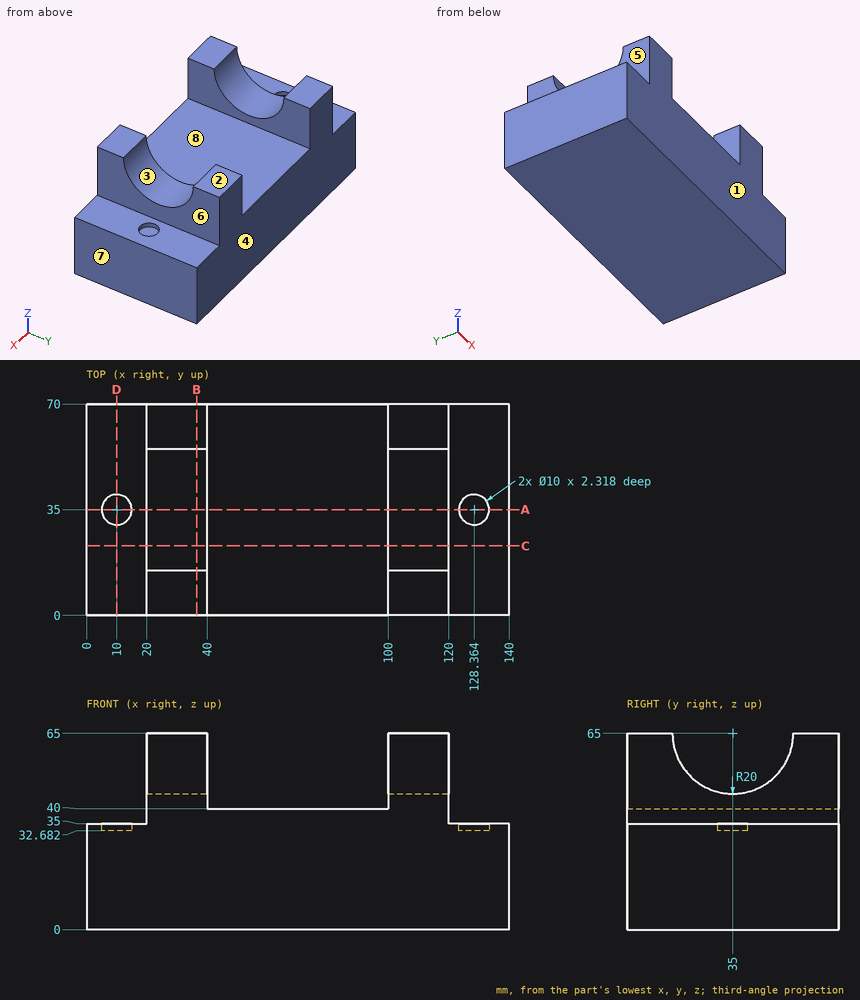
Here's the drawing with two shaded views (mm, measured from the low corner). I have some questions. A direction names the side the tool comes from. Round coordinates to 2 decimals unless told otherwise and drop trailing zeros. Write each loop counter-clockwise with the first axis right and the second up, starting at its lowest first coordinate (ties: lowest second). Pieces come first, ordered by that corner, then holes. Notation, with made-up numbers: M 50,50 L 71,50 A32 ccw 71,82 Z; hole C 4,69.5 d10. An arc over 180 degrees is marked long. Answer in a Markdown table with one row per item. Add a question column.
Q1. On a 3-axis mill with a long thin cutter (end or side, diameter ignored), from which of +Z, -Z, +X, -X, +Y, -Y can I reach the whole of each face in a straight line? I mean the marked faces 5, 6, 7 and 8. Say none if no direction works.
Q2. Imagine slicing it at A-A (y = 35). Please give me the cut outline in (x, z), then the cut area to 3 significant figures.
Q3. If we mould it in two halves opening along Y, with no side actions, what happens to the marked faces 1, 2, 3 and 4? For each: +Y half, -Y half, draft (parallel to the pull), parting line (faces both ways), or undercut.
Q4. If I drill on line 1 (X direction, y = 45, z = 46); line 2 (Y direction, x = 10, z = 33.65); line 3 (Z direction, x = 62.5, y = 61.5), over which ranges is the centre line in solid material (lowest first)? Write a range as from..to.
Q5. Imagine slicing it at C-C (y = 23). Please give me the cut outline in (x, z), then the cut area to 3 significant figures.
Q6. Imagine slicing it at B-B (x = 36.5). Please give me the cut outline in (y, z), then the cut area to 3 significant figures.
Q7. Will these pins go through, and if not, where does the flat tip stop? pin 1 Ø16 at (x, y) = (130.5, 28.5) entering from +Z; pin 2 Ø12 at (x, y) = (90, 61.5) entering from +Z; pin 3 Ø12 at (x, y) = (102, 28.5) entering from +Z; pin 4 Ø1 at (y, z) = (60.5, 11) entering from -X.
Q8. Imagine slicing it at D-D (x = 10). Please give me the cut outline in (y, z).
Values:
| question | item | result |
|---|---|---|
| 1 | face 5 | +Z, -X, +Y, -Y |
| 1 | face 6 | +Z, +X, +Y, -Y |
| 1 | face 7 | +Z, -Z, +X, +Y, -Y |
| 1 | face 8 | +Z, +Y, -Y |
| 2 | outline | M 0,0 L 140,0 L 140,35 L 133.36,35 L 133.36,32.68 L 123.36,32.68 L 123.36,35 L 120,35 L 120,45 L 100,45 L 100,40 L 40,40 L 40,45 L 20,45 L 20,35 L 15,35 L 15,32.68 L 5,32.68 L 5,35 L 0,35 Z |
| 2 | area | 5,550 mm^2 |
| 3 | face 1 | -Y half |
| 3 | face 2 | draft |
| 3 | face 3 | undercut |
| 3 | face 4 | +Y half |
| 4 | line 1 | 20..40, 100..120 |
| 4 | line 2 | 0..30, 40..70 |
| 4 | line 3 | 0..40 |
| 5 | outline | M 0,0 L 140,0 L 140,35 L 120,35 L 120,49 L 100,49 L 100,40 L 40,40 L 40,49 L 20,49 L 20,35 L 0,35 Z |
| 5 | area | 5,760 mm^2 |
| 6 | outline | M 0,0 L 70,0 L 70,65 L 55,65 A20 cw 15,65 L 0,65 Z |
| 6 | area | 3,920 mm^2 |
| 7 | pin 1 | z = 35 |
| 7 | pin 2 | z = 40 |
| 7 | pin 3 | z = 49.39 |
| 7 | pin 4 | x = 0 |
| 8 | outline | M 0,0 L 70,0 L 70,35 L 40,35 L 40,32.68 L 30,32.68 L 30,35 L 0,35 Z |
